Design review of the part built by this model. Coordinates are the model's own, in mm. Coordinates: 2 decimals unless noted, no trailing zeros. Loops run counter-clockwise (first coordinate to the right, second up) from the corner with the lowest first, then second, coordinate; pieces in that order, holes last. Notation, with made-up numbers: (43, 89.5) - (76, 89.5) arc R9 cw to (76, 99.5) - close; hole circle Ø5 at (76, 53.25). An arc over 180 degrees is marked (long way). Answer in a Markdown table with one row per item. Add a question column.
(1) To check wall thickness, follow L1, parallel to Y at x = -25.45, z = 1.6; L2, parallel to X at y = -6, z = 1.1; L3, parallel to Y at x = -29.5, z = 0.8. State the ranges of each line that lie inside material, in increasing order. Write a range as [from, to].
(2) We need section D-D, the plane x = -5.5. Write out the cut boundary in (y, z), plus the area to 3 significant figures.
(3) Clearance check with flat-ended pins moving along their axes: pin 1 (0.6 mm diameter, centred on y = -23, z = 1, fed in from +X); pin 2 (0.6 mm diameter, centred on y = -10.5, z = 0.5, fed in from -X); pin 3 (0.6 mm diameter, centred on x = -15, z = 1, fed in from -Y); pin 4 (5 mm diameter, centred on x = -22.5, y = -19.5, fed in from -Z). State where each tip first meets the part, or that it passes through.
(4) We need section B-B, the plane x = -21.5. Write out the cut boundary in (y, z).
(5) We need section C-C, the plane z = 1.4. Give the number of separate pieces and of enclosed holes in the cut face, plus the area to 3 significant figures.
(6) We need section A-A, the plane y = -7. Write out the cut boundary in (x, z), plus the area to 3 significant figures.
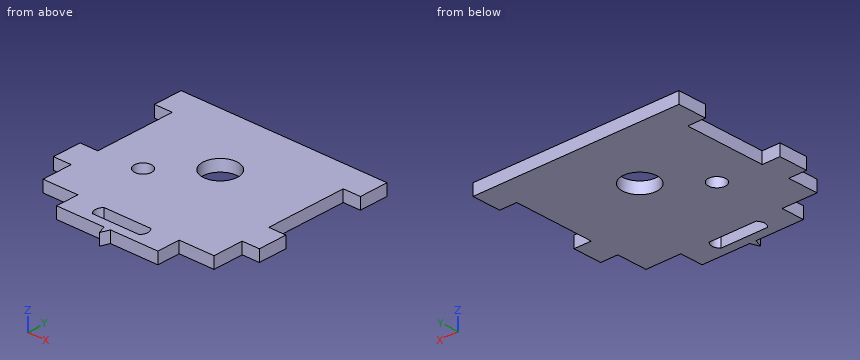
from build123d import *

# Parameters (mm, degrees)
SKETCH_1_R      = 3
SKETCH_1_R_2    = 1.5
EXTRUDE_1_DEPTH = 2


with BuildPart() as part:
    # 草图1 → 凸台-拉伸1 (new body)
    with BuildSketch(Plane.XY):
        Polygon((0, 0), (0, 5), (-3, 5), (-33, 5), (-36, 5), (-36, 0), (-33, 0), (-32.9, 0), (-32.9, -14), (-33, -14), (-36, -14), (-36, -19), (-33, -19), (-32.9, -19), (-32.9, -24.3), (-26.8, -24.3), (-26.8, -28.3), (-18.511559339, -28.3), (-17.95, -29.8), (-17.388440661, -28.3), (-9.1, -28.3), (-9.1, -24.3), (-3, -24.3), (-3, -19), (0, -19), (0, -14), (-3, -14), (-3, 0), align=None)
        with Locations((-18, -7)):
            Circle(SKETCH_1_R, mode=Mode.SUBTRACT)
        with Locations((-25.45, -13.5)):
            Circle(SKETCH_1_R_2, mode=Mode.SUBTRACT)
        with BuildLine():
            Line((-22.05, -24.5), (-13.85, -24.5))
            ThreePointArc((-13.85, -24.5), (-13.394365081, -25.6), (-13.85, -26.7))
            Line((-13.85, -26.7), (-22.05, -26.7))
            ThreePointArc((-22.05, -26.7), (-22.505634919, -25.6), (-22.05, -24.5))
        make_face(mode=Mode.SUBTRACT)
    extrude(amount=EXTRUDE_1_DEPTH)


solid = part.part
Responses:
| question | item | result |
|---|---|---|
| 1 | L1 | y = [-28.3, -15], [-12, 5] |
| 1 | L2 | x = [-32.9, -20.83], [-15.17, -3] |
| 1 | L3 | y = [-24.3, 5] |
| 2 | outline | (-24.3, 0) - (5, 0) - (5, 2) - (-24.3, 2) - close |
| 2 | area | 58.6 mm2 |
| 3 | pin 1 | stops at x = -3 |
| 3 | pin 2 | stops at x = -32.9 |
| 3 | pin 3 | stops at y = -28.3 |
| 3 | pin 4 | stops at z = 0 |
| 4 | outline | (-28.3, 0) - (-26.7, 0) - (-26.7, 2) - (-28.3, 2) - close; (-24.5, 0) - (5, 0) - (5, 2) - (-24.5, 2) - close |
| 5 | separate pieces | 1 |
| 5 | enclosed holes | 3 |
| 5 | area | 954 mm2 |
| 6 | outline | (-32.9, 0) - (-21, 0) - (-21, 2) - (-32.9, 2) - close; (-15, 0) - (-3, 0) - (-3, 2) - (-15, 2) - close |
| 6 | area | 47.8 mm2 |
